Model file for the job. Use its own axes, mm. Face numbers are marked on the shaded views. Give positions to 0.01 mm unless a question says otherwise; leave off trailing zeros. Write each loop counter-clockwise with the first axis right and the second up, starting at its lowest first coordinate (ties: lowest second). Pieces come first, ordered by that corner, then holes.
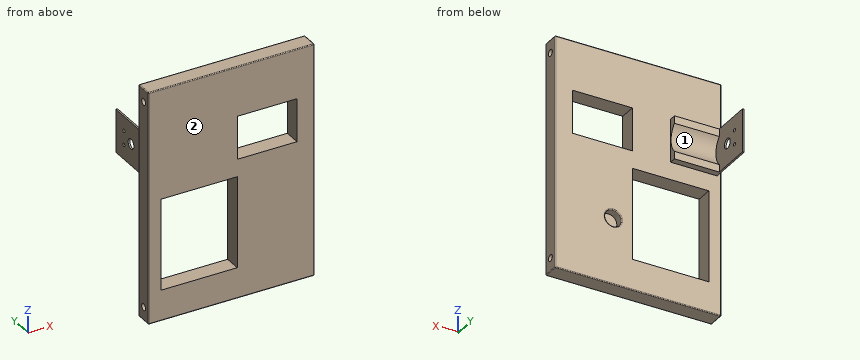
```python
from build123d import *

# Parameters (mm, degrees)
SKETCH2_W               = 100
SKETCH2_H               = 140
BOSS_EXTRUDE1_DEPTH     = 10
SKETCH3_R               = 5
MOUNTHOLE_DEPTH         = 5
SKETCH4_R               = 2
CUT_EXTRUDE2_DEPTH      = 101
SKETCH5_R               = 2
CUT_EXTRUDE3_DEPTH      = 101
FILLET4_R               = 0.5
FILLET6_R               = 0.5
SKETCH7_W               = 28
SKETCH7_H               = 26
BOSS_EXTRUDE2_DEPTH     = 4
SKETCH21_W              = 46
SKETCH21_H              = 55
SKETCH21_W_2            = 36
SKETCH21_H_2            = 26
CUT_EXTRUDE10_DEPTH     = 11
SKETCH10_W              = 1
SKETCH10_H              = 26
BOSS_EXTRUDE3_DEPTH     = 24
SKETCH13_R              = 3
SKETCH13_R_2            = 1
CUT_EXTRUDE6_DEPTH      = 1
CUT_EXTRUDE9_DEPTH      = 70.5
CUT_EXTRUDE9_DEPTH_BACK = 27


with BuildPart() as part:
    # Sketch2 → Boss-Extrude1 (new body)
    with BuildSketch(Plane(origin=(0, 0, 0), x_dir=(1, 0, 0), z_dir=(0, 1, 0))):
        with Locations((50, 70)):
            Rectangle(SKETCH2_W, SKETCH2_H)
    extrude(amount=BOSS_EXTRUDE1_DEPTH)

    # Sketch3 → MountHole (cut)
    with BuildSketch(Plane(origin=(0, 10, 0), x_dir=(1, 0, 0), z_dir=(0, 1, 0))):
        with Locations((65, 100)):
            Circle(SKETCH3_R)
    extrude(amount=-MOUNTHOLE_DEPTH, mode=Mode.SUBTRACT)

    # Sketch4 → Cut-Extrude2 (cut, through all)
    with BuildSketch(Plane.ZY):
        with Locations((-8, 5)):
            Circle(SKETCH4_R)
    extrude(amount=-CUT_EXTRUDE2_DEPTH, mode=Mode.SUBTRACT)

    # Sketch5 → Cut-Extrude3 (cut, through all)
    with BuildSketch(Plane.ZY):
        with Locations((-132, 5)):
            Circle(SKETCH5_R)
    extrude(amount=-CUT_EXTRUDE3_DEPTH, mode=Mode.SUBTRACT)

    # Fillet4
    fillet4_edges = [part.edges().sort_by_distance(p)[0] for p in [
        (50, 10, -140),
        (0, 10, -70),
        (50, 10, 0),
        (0, 0, -70),
        (50, 0, -140),
        (100, 0, -70),
        (50, 0, 0),
        (0, 5, 0),
        (0, 5, -140),
        (100, 5, -140),
        (100, 5, 0),
        (100, 10, -70),
    ]]
    fillet(fillet4_edges, radius=FILLET4_R)

    # Fillet6
    fillet6_edges = [part.edges().sort_by_distance(p)[0] for p in [
        (60, 10, -100),
    ]]
    fillet(fillet6_edges, radius=FILLET6_R)

    # Sketch7 → Boss-Extrude2 (add)
    with BuildSketch(Plane(origin=(0, 10, 0), x_dir=(1, 0, 0), z_dir=(0, 1, 0))):
        with Locations((16.5, 43)):
            Rectangle(SKETCH7_W, SKETCH7_H)
    extrude(amount=BOSS_EXTRUDE2_DEPTH)

    # Sketch21 → Cut-Extrude10 (cut, through all)
    with BuildSketch(Plane(origin=(0, 10, 0), x_dir=(1, 0, 0), z_dir=(0, 1, 0))):
        with Locations((30.5, 94)):
            Rectangle(SKETCH21_W, SKETCH21_H)
        with Locations((71.5, 43)):
            Rectangle(SKETCH21_W_2, SKETCH21_H_2)
    extrude(amount=-CUT_EXTRUDE10_DEPTH, mode=Mode.SUBTRACT)

    # Sketch10 → Boss-Extrude3 (add)
    with BuildSketch(Plane(origin=(0, 14, 0), x_dir=(1, 0, 0), z_dir=(0, 1, 0))):
        with Locations((3, 43)):
            Rectangle(SKETCH10_W, SKETCH10_H)
    extrude(amount=BOSS_EXTRUDE3_DEPTH)

    # Sketch13 → Cut-Extrude6 (cut)
    with BuildSketch(Plane.ZY.offset(-2.5)):
        with Locations((-43, 22.354)):
            Circle(SKETCH13_R)
        with Locations((-38.75, 29.715215932)):
            Circle(SKETCH13_R_2)
        with Locations((-47.25, 29.715215932)):
            Circle(SKETCH13_R_2)
    extrude(amount=-CUT_EXTRUDE6_DEPTH, mode=Mode.SUBTRACT)

    # Sketch20 → Cut-Extrude9 (cut, two sides)
    with BuildSketch(Plane(origin=(30.5, 0, 0), x_dir=(0, 0, -1), z_dir=(1, 0, 0))) as cut_extrude9_sk:
        with BuildLine():
            Line((-205.175487121, 14), (30, 14))
            Line((30, 14), (34.519834012, 14))
            ThreePointArc((34.519834012, 14), (43, 10.490393679), (51.480165988, 14))
            Line((51.480165988, 14), (56, 14))
            Line((56, 14), (291.175487121, 14))
            Line((291.175487121, 14), (291.175487121, 484.350974241))
            Line((291.175487121, 484.350974241), (-205.175487121, 484.350974241))
            Line((-205.175487121, 484.350974241), (-205.175487121, 14))
        make_face()
    extrude(amount=CUT_EXTRUDE9_DEPTH, mode=Mode.SUBTRACT)
    extrude(cut_extrude9_sk.sketch, amount=-CUT_EXTRUDE9_DEPTH_BACK, mode=Mode.SUBTRACT)


solid = part.part
```
1. Slice it at D-D, the plane z = -8. Write the cut outline in (x, y).
Calculated:
outline: (0, 0.5) arc R0.5 ccw to (0.5, 0) - (99.5, 0) arc R0.5 ccw to (100, 0.5) - (100, 3) - (0, 3) - close; (0, 7) - (100, 7) - (100, 9.5) arc R0.5 ccw to (99.5, 10) - (0.5, 10) arc R0.5 ccw to (0, 9.5) - close
2. Slice it at A-A, the plane x = 55. Write the cut outline in (y, z), and give its area (3 significant figures).
Calculated:
outline: (0, -139.5) arc R0.5 ccw to (0.5, -140) - (9.5, -140) arc R0.5 ccw to (10, -139.5) - (10, -56) - (0, -56) - close; (0, -30) - (10, -30) - (10, -0.5) arc R0.5 ccw to (9.5, 0) - (0.5, 0) arc R0.5 ccw to (0, -0.5) - close; hole circle Ø4 at (5, -132); hole circle Ø4 at (5, -8)
area: 1,110 mm2
3. Pull direction Z, two halves, no side cores. Call the marked faces 1 and 2: +Z half, -Z half, draft (parallel to the pull), parting line (faces both ways), or undercut.
Calculated:
face 1: undercut
face 2: draft
4. Probe probe 1 along X at (y, z) = (7.35, -100); probe 2 along Z at (x, y) = (18, 3.5); probe 3 along Y at (x, z) = (3.2, -38.75). List the from-to ranges inside material, lowest first.
Calculated:
probe 1: x = 0 to 7.5, 53.5 to 60, 70 to 100
probe 2: z = -140 to -133.32, -130.68 to -121.5, -66.5 to -9.32, -6.68 to 0
probe 3: y = 0 to 28.72, 30.72 to 38
5. Slice it at C-C, the plane x = 92.5. Write the cut outline in (y, z).
Calculated:
outline: (0, -139.5) arc R0.5 ccw to (0.5, -140) - (9.5, -140) arc R0.5 ccw to (10, -139.5) - (10, -0.5) arc R0.5 ccw to (9.5, 0) - (0.5, 0) arc R0.5 ccw to (0, -0.5) - close; hole circle Ø4 at (5, -132); hole circle Ø4 at (5, -8)
6. Slice it at B-B, the plane z = -100. Write the cut outline in (x, y).
Calculated:
outline: (0, 0.5) arc R0.5 ccw to (0.5, 0) - (7.5, 0) - (7.5, 10) - (0.5, 10) arc R0.5 ccw to (0, 9.5) - close; (53.5, 0) - (99.5, 0) arc R0.5 ccw to (100, 0.5) - (100, 9.5) arc R0.5 ccw to (99.5, 10) - (70.5, 10) arc R0.5 ccw to (70, 9.5) - (70, 5) - (60, 5) - (60, 9.5) arc R0.5 ccw to (59.5, 10) - (53.5, 10) - close
7. Pin check, flat tips, straight feed: P1, Ø8, axis at y = 5.5, z = -39.5, coming from the -X side; P2, Ø3, axis at x = 63, z = -98, coming from the +Y side; P3, Ø3.5, axis at x = 20, z = -31.5, coming from the +Y side; P4, Ø8, axis at y = 21, z = -28.5, coming from the +X side. Stop position of each tip, or through.
Calculated:
P1: stops at x = 0
P2: stops at y = 5
P3: stops at y = 14
P4: stops at x = 3.5
